Work out the finished part from the listing and answer in its coordinate system (mm). A direction names the side the tool comes from. Give positions to 0.01 mm unless a question says otherwise; leave off trailing zeros. Loops run counter-clockwise (first coordinate to the right, second up) from the corner with the lowest first, then second, coordinate; pieces in that order, holes last. Notation, with made-up numbers: (7, 31) - (23, 31) arc R23 cw to (23, 67) - close; hole circle Ø8 at (45.5, -38). An arc over 180 degrees is marked (long way). Use one line per item in the form item = value. Start each with the question number.
from build123d import *

# Parameters (mm, degrees)
F1_DEPTH = 3.175
F2_R     = 0.3175
F3_R     = 0.3175


with BuildPart() as f1:
    # F0 (on Front) → F1 (new body)
    with BuildSketch(Plane.XZ):
        with BuildLine():
            ThreePointArc((-19.05, -21.065116), (-18.120064, -23.31018), (-15.875, -24.240116))
            Line((-15.875, -24.240116), (15.875, -24.240116))
            ThreePointArc((15.875, -24.240116), (18.120064, -23.31018), (19.05, -21.065116))
            Line((19.05, -21.065116), (19.05, -11.025942))
            ThreePointArc((19.05, -11.025942), (18.120064, -8.780878), (15.875, -7.850942))
            Line((15.875, -7.850942), (1.27, -7.850942))
            ThreePointArc((1.27, -7.850942), (-3.220128, -5.99107), (-5.08, -1.500942))
            Line((-5.08, -1.500942), (-5.08, 9.852602))
            ThreePointArc((-5.08, 9.852602), (0, 14.932602), (5.08, 9.852602))
            Line((5.08, 9.852602), (5.08, 4.849058))
            ThreePointArc((5.08, 4.849058), (5.823949, 3.053007), (7.62, 2.309058))
            Line((7.62, 2.309058), (15.875, 2.309058))
            ThreePointArc((15.875, 2.309058), (18.120064, 3.238994), (19.05, 5.484058))
            Line((19.05, 5.484058), (19.05, 24.518112))
            ThreePointArc((19.05, 24.518112), (18.790355, 26.490313), (18.029114, 28.328112))
            Line((18.029114, 28.328112), (6.599114, 48.125452))
            ThreePointArc((6.599114, 48.125452), (0, 51.935452), (-6.599114, 48.125452))
            Line((-6.599114, 48.125452), (-18.624631, 27.296646))
            ThreePointArc((-18.624631, 27.296646), (-18.941814, 26.530896), (-19.05, 25.709146))
            Line((-19.05, 25.709146), (-19.05, -21.065116))
        make_face()
    extrude(amount=F1_DEPTH)

    # F2
    f2_edges = [f1.edges().sort_by_distance(p)[0] for p in [
        (19.05, -3.175, -16.045529),
        (18.120064, -3.175, -8.780878),
        (8.5725, -3.175, -7.850942),
        (-3.220128, -3.175, -5.99107),
        (-5.08, -3.175, 4.17583),
        (0, -3.175, 14.932602),
        (5.08, -3.175, 7.35083),
        (5.823949, -3.175, 3.053007),
        (11.7475, -3.175, 2.309058),
        (18.120064, -3.175, 3.238994),
        (19.05, -3.175, 15.001085),
        (18.790355, -3.175, 26.490313),
        (12.314114, -3.175, 38.226782),
        (0, -3.175, 51.935452),
        (-12.611872, -3.175, 37.711049),
        (-18.941814, -3.175, 26.530896),
        (-19.05, -3.175, 2.322015),
        (-18.120064, -3.175, -23.31018),
        (0, -3.175, -24.240116),
        (18.120064, -3.175, -23.31018),
    ]]
    fillet(f2_edges, radius=F2_R)

    # F3
    f3_edges = [f1.edges().sort_by_distance(p)[0] for p in [
        (19.05, 0, -16.045529),
        (18.120064, 0, -8.780878),
        (8.5725, 0, -7.850942),
        (-3.220128, 0, -5.99107),
        (-5.08, 0, 4.17583),
        (0, 0, 14.932602),
        (5.08, 0, 7.35083),
        (5.823949, 0, 3.053007),
        (11.7475, 0, 2.309058),
        (18.120064, 0, 3.238994),
        (19.05, 0, 15.001085),
        (18.790355, 0, 26.490313),
        (12.314114, 0, 38.226782),
        (0, 0, 51.935452),
        (-12.611872, 0, 37.711049),
        (-18.941814, 0, 26.530896),
        (-19.05, 0, 2.322015),
        (-18.120064, 0, -23.31018),
        (0, 0, -24.240116),
        (18.120064, 0, -23.31018),
    ]]
    fillet(f3_edges, radius=F3_R)


solid = f1.part
1) Flat-ended cylindrical pins translate along their axes: pin 1 Ø1.3 at (x, y) = (6, -1.5) entering from +Z; pin 2 Ø1 at (x, y) = (2, -1) entering from +Z. Find the tip coordinate at first contact, or state that the pin passes through.
2) A tool of negligible diameter and unlimited length cuts with its end or side. For faces 5 (the flat face through (-5.08, -2, 4)), 6 (the cylindrical face through (12.15, -0.09, 38.32)), 7 (the cylindrical face through (18.145, -1.57, -8.806)), from which of +Z, -Z, +X, -X, +Y, -Y can it reach the whole face along a straight path? Write none if from no direction.
3) Determine the mould class of faces 1 (the cylindrical face through (-0.11, -1.57, 14.93)), 2 (the flat face through (19.05, -2, -16)), 3 (the cylindrical face through (18.8, -1.57, 26.46)), 4 (the flat face through (5.08, -2, 7)) for opening direction Z: released by +Z, released by -Z, zero draft, split by the parting line, or undercut.
4) A cutting plane is placed at A-A (y = -2.2). Give the vertices of the cut face in (x, z) (3 decimals), plus the area to 3 significant figures.
5) Find the intervals of material crossed by probe 1 along X at (y, z) = (-2.1, -1); probe 2 along Z at (x, y) = (1, -1.3); probe 3 along Z at (x, y) = (14, -0.9), in increasing order.
Answer sheet:
q1.pin_1 = 49.74
q1.pin_2 = 51.79
q2.face_5 = +Y, -Y
q2.face_6 = +Z, +X, +Y
q2.face_7 = +X, +Y, -Y
q3.face_1 = undercut
q3.face_2 = zero draft
q3.face_3 = released by +Z
q3.face_4 = undercut
q4.outline = (-19.05, -21.065) arc R3.175 ccw to (-15.875, -24.24) - (15.875, -24.24) arc R3.175 ccw to (19.05, -21.065) - (19.05, -11.026) arc R3.175 ccw to (15.875, -7.851) - (1.27, -7.851) arc R6.35 cw to (-5.08, -1.501) - (-5.08, 9.853) arc R5.08 cw to (5.08, 9.853) - (5.08, 4.849) arc R2.54 ccw to (7.62, 2.309) - (15.875, 2.309) arc R3.175 ccw to (19.05, 5.484) - (19.05, 24.518) arc R7.62 ccw to (18.029, 28.328) - (6.599, 48.125) arc R7.62 ccw to (-6.599, 48.125) - (-18.625, 27.297) arc R3.175 ccw to (-19.05, 25.709) - close
q4.area = 2,160 mm²
q5.probe_1 = -19.05 to -5.08
q5.probe_2 = -24.24 to -7.85, 14.83 to 51.87
q5.probe_3 = -24.24 to -7.85, 2.31 to 35.31
